```python
from build123d import *

# Parameters (mm, degrees)
SKETCH1_R               = 4.255
BOSS_EXTRUDE3_DEPTH     = 5
BOSS_EXTRUDE3_2_DEPTH   = 5
BOSS_EXTRUDE7_START     = -5
BOSS_EXTRUDE7_DEPTH     = 1.5
CUT_EXTRUDE1_DEPTH      = 15.896343511
CUT_EXTRUDE1_DEPTH_BACK = 15.896343511
SKETCH2_R               = 2.5


with BuildPart() as part:
    # Sketch1 → Boss-Extrude3 (new, symmetric)
    with BuildSketch(Plane.XY):
        with Locations((6.35, 0)):
            Circle(SKETCH1_R)
    extrude(amount=BOSS_EXTRUDE3_DEPTH, both=True)



with BuildPart() as body_2:
    # Sketch1 → Boss-Extrude3 2 (new, symmetric)
    with BuildSketch(Plane.XY):
        with Locations((-6.35, 0)):
            Circle(SKETCH1_R)
    extrude(amount=BOSS_EXTRUDE3_2_DEPTH, both=True)


with BuildPart() as part_1:
    add(part.part)

    add(body_2.part)  # Boss-Extrude7 merges body 2
    # Sketch1_5 → Boss-Extrude7 (add)
    with BuildSketch(Plane.XY.offset(BOSS_EXTRUDE7_START)):
        with BuildLine():
            ThreePointArc((-3.26499838, 4.858270268), (-12.105, 0), (-3.26499838, -4.858270268))
            ThreePointArc((-3.26499838, -4.858270268), (0, -3.909220161), (3.26499838, -4.858270268))
            ThreePointArc((3.26499838, -4.858270268), (12.105, 0), (3.26499838, 4.858270268))
            ThreePointArc((3.26499838, 4.858270268), (0, 3.909220161), (-3.26499838, 4.858270268))
        make_face()
    boss_extrude7 = extrude(amount=-BOSS_EXTRUDE7_DEPTH)

    # Mirror1: Boss-Extrude7 across plane
    add(boss_extrude7.mirror(Plane.XY))

    # Sketch2 → Cut-Extrude1 (cut, two sides: drawn at the far end of the back side and taken through both)
    with BuildSketch(Plane.XY.offset(-CUT_EXTRUDE1_DEPTH_BACK)):
        with Locations((-6.35, 0)):
            Circle(SKETCH2_R)
        with Locations(Location((6.35, 0, 0), (0, 0, 180))):
            Circle(SKETCH2_R)
    extrude(amount=CUT_EXTRUDE1_DEPTH + CUT_EXTRUDE1_DEPTH_BACK, mode=Mode.SUBTRACT)


solid = part_1.part
```
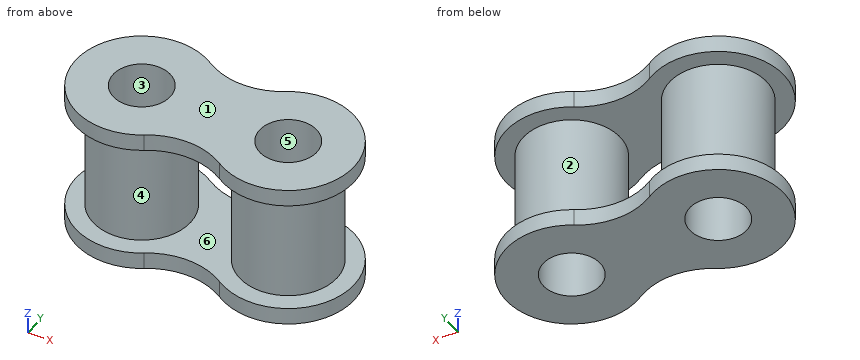
Geometry: final body of the model. Coordinates: model frame, mm. Face numbers are marked on the shaded views. A direction names the side the tool comes from. Coordinates: 2 decimals unless noted, no trailing zeros. Order: outer loops, then holes, each group sorted by start corner. A loop starts at its lowest first (then second) coordinate and runs counter-clockwise, first axis right, second up. Notation, with made-up numbers: (22.5, 44) -> (42.5, 44) arc R21 cw to (42.5, 61) -> close; hole circle Ø6 at (-1.5, -32). An arc over 180 degrees is marked (long way). Answer in a Markdown table with one row per item.
Item 1: Contact query for flat-ended pins moving along their axis: P1, Ø2, axis at x = -1.5, z = -1.5, coming from the +Y side; P2, Ø4, axis at x = -1.5, z = 1.5, coming from the +Y side; P3, Ø4, axis at y = 1.5, z = 1, coming from the +X side (3 decimals). Output: stop coordinate, or through.
Return value:
| item | result |
|---|---|
| P1 | stops at y = 1.81 |
| P2 | stops at y = 3.16 |
| P3 | stops at x = 10.605 |
Item 2: Access query for the marked faces 5 and 6. Directions: +Z, -Z, +X, -X, +Y, -Y. A direction counts if a zero-diameter tool reaches every point of the face in a straight line with its end or side. Return the directions, or none.
Return value:
| item | result |
|---|---|
| face 5 | +Z, -Z |
| face 6 | none |
Item 3: Ray query, L1, parallel to Z at x = -4, y = 5; L2, parallel to Y at x = -6.35, z = 2 (3 decimals); L3, parallel to X at y = 1.75, z = -1.5. Return the intervals inside material, ascending.
Return value:
| item | result |
|---|---|
| L1 | z = -6.5 to -5, 5 to 6.5 |
| L2 | y = -4.255 to -2.5, 2.5 to 4.255 |
| L3 | x = -10.23 to -8.14, -4.56 to -2.47, 2.47 to 4.56, 8.14 to 10.23 |
Item 4: Draft query along Z for the marked faces 1, 2, 3 and 4. Return one class per face: released by +Z, released by -Z, zero draft, split by the parting line, or undercut.
Return value:
| item | result |
|---|---|
| face 1 | released by +Z |
| face 2 | undercut |
| face 3 | zero draft |
| face 4 | undercut |
Item 5: Section C-C on z = -3. Output: boundary loops of the cut face in (x, y) (3 decimals), plus the area to 3 significant figures.
Return value:
| item | result |
|---|---|
| outline | circle Ø8.51 at (-6.35, 0); circle Ø8.51 at (6.35, 0); hole circle Ø5 at (-6.35, 0); hole circle Ø5 at (6.35, 0) |
| area | 74.5 mm² |
Item 6: Section B-B on x = 6.35. Output: boundary loops of the cut face in (y, z) (3 decimals), plus the area to 3 significant figures.
Return value:
| item | result |
|---|---|
| outline | (-5.755, -6.5) -> (-2.5, -6.5) -> (-2.5, 6.5) -> (-5.755, 6.5) -> (-5.755, 5) -> (-4.255, 5) -> (-4.255, -5) -> (-5.755, -5) -> close; (2.5, -6.5) -> (5.755, -6.5) -> (5.755, -5) -> (4.255, -5) -> (4.255, 5) -> (5.755, 5) -> (5.755, 6.5) -> (2.5, 6.5) -> close |
| area | 54.6 mm² |
Item 7: Section D-D on y = -1.5. Output: boundary loops of the cut face in (x, z), plus the area to 3 significant figures.
Return value:
| item | result |
|---|---|
| outline | (-11.91, -6.5) -> (-8.35, -6.5) -> (-8.35, 6.5) -> (-11.91, 6.5) -> (-11.91, 5) -> (-10.33, 5) -> (-10.33, -5) -> (-11.91, -5) -> close; (-4.35, -6.5) -> (4.35, -6.5) -> (4.35, 6.5) -> (-4.35, 6.5) -> close; (8.35, -6.5) -> (11.91, -6.5) -> (11.91, -5) -> (10.33, -5) -> (10.33, 5) -> (11.91, 5) -> (11.91, 6.5) -> (8.35, 6.5) -> close; hole (-2.37, -5) -> (2.37, -5) -> (2.37, 5) -> (-2.37, 5) -> close |
| area | 127 mm² |
Item 8: Section A-A on y = 0. Output: boundary loops of the cut face in (x, z) (3 decimals), plus the area to 3 significant figures.
Return value:
| item | result |
|---|---|
| outline | (-12.105, -6.5) -> (-8.85, -6.5) -> (-8.85, 6.5) -> (-12.105, 6.5) -> (-12.105, 5) -> (-10.605, 5) -> (-10.605, -5) -> (-12.105, -5) -> close; (-3.85, -6.5) -> (3.85, -6.5) -> (3.85, 6.5) -> (-3.85, 6.5) -> close; (8.85, -6.5) -> (12.105, -6.5) -> (12.105, -5) -> (10.605, -5) -> (10.605, 5) -> (12.105, 5) -> (12.105, 6.5) -> (8.85, 6.5) -> close; hole (-2.095, -5) -> (2.095, -5) -> (2.095, 5) -> (-2.095, 5) -> close |
| area | 113 mm² |
